Input: part model. Units: mm. Frame: model coordinates. A direction names the side the tool comes from. Coordinates: 2 decimals unless noted, no trailing zeros. Loops run counter-clockwise (first coordinate to the right, second up) from the corner with the lowest first, then second, coordinate; pieces in that order, holes last.
(1) Mould query, pull axis X, two halves, no side actions, for faces 6 (the face through (0, 4, -10)), 7 (the face through (22.5, 5, -10.1)), 8 (the face through (5, 1, -10)), 9 (the face through (45, 4, -10)). Classes: released by +X, released by -X, zero draft, split by the parting line, or undercut.
(2) Contact query for flat-ended pins moving along their axis: P1, Ø3.5, axis at x = 8, z = -8, coming from the -Y side; P2, Ø2.5, axis at x = 37.5, z = -11, coming from the -Y side. Output: stop coordinate, or through.
(3) Section B-B, the plane z = -10. Return loops of the section in (x, y), then the cut area to 3 significant figures.
(4) Set-up query: faces 1 (the face through (5, 0.5, -2.8)), 2 (the face through (2.7, 0.5, -5.5)), 3 (the face through (44.715, 0.301, -17.288)), 4 (the face through (24, 1, -14.5)), 5 (the face through (29, 0, -17)). Return all of +Z, -Z, +X, -X, +Y, -Y with unobstructed straight access to the full face (end or side cutting, diameter ignored); none if empty.
(5) Section C-C, the plane x = 8.5. Return loops of the section in (y, z), then the cut area to 3 significant figures.
(6) Section A-A, the plane y = 5. Return loops of the section in (x, z).
(7) Line query: L1, parallel to Z at x = 23.5, y = 1.75; L2, parallel to Z at x = 6.5, y = 7; L3, parallel to X at y = 5.25, z = -7. Output: solid intervals per line, ascending.
```python
from build123d import *
from OCP.BRepFilletAPI import BRepFilletAPI_MakeChamfer

# Parameters (mm, degrees)
SKETCH_1_W          = 45
SKETCH_1_H          = 20
EXTRUDE_1_DEPTH     = 8
CUT_EXTRUDE_1_DEPTH = 2
CUT_EXTRUDE_2_DEPTH = 1
CHAMFER_1_SIZE      = 1
CHAMFER_2_SIZE      = 1
CHAMFER_2_SIZE_2    = 1.732050808
FILLET_1_R          = 1


with BuildPart() as part:
    # 草图1 → 凸台-拉伸1 (new body)
    with BuildSketch(Plane(origin=(0, 0, 0), x_dir=(1, 0, 0), z_dir=(0, 1, 0))):
        with Locations((22.5, 10)):
            Rectangle(SKETCH_1_W, SKETCH_1_H)
        with BuildLine():
            Line((18, 5.5), (10, 5.5))
            ThreePointArc((10, 5.5), (5.5, 10), (10, 14.5))
            Line((10, 14.5), (18, 14.5))
            ThreePointArc((18, 14.5), (22.5, 10), (18, 5.5))
        make_face(mode=Mode.SUBTRACT)
    extrude(amount=EXTRUDE_1_DEPTH)

    # 草图2 → 切除-拉伸1 (cut)
    with BuildSketch(Plane.XZ):
        with BuildLine():
            Line((45, -5.5), (45, -14.5))
            Line((45, -14.5), (10, -14.5))
            ThreePointArc((10, -14.5), (5.5, -10), (10, -5.5))
            Line((10, -5.5), (45, -5.5))
        make_face()
    extrude(amount=-CUT_EXTRUDE_1_DEPTH, mode=Mode.SUBTRACT)

    # 草图3 → 切除-拉伸2 (cut)
    with BuildSketch(Plane.XZ):
        Polygon((0, -5.5), (5.5, -5.5), (5.5, 0), (12.1, 0), (12.1, -20), (5.5, -20), (5.5, -14.5), (0, -14.5), align=None)
    extrude(amount=-CUT_EXTRUDE_2_DEPTH, mode=Mode.SUBTRACT)

    # 倒角1
    chamfer_1_edges = [part.edges().sort_by_distance(p)[0] for p in [
        (0, 0, -17.25),
        (5.5, 0, -17.25),
        (5.5, 0, -2.75),
        (0, 0, -2.75),
    ]]
    chamfer(chamfer_1_edges, length=CHAMFER_1_SIZE - 0.0001)  # a hair under: the kernel refuses the full size

    # 倒角2
    chamfer_2_edges_1 = [part.edges().sort_by_distance(p)[0] for p in [
        (12.1, 0, -17.25),
    ]]
    chamfer_2_side_1 = [part.faces().sort_by_distance(p)[0] for p in [
        (12.1, 0.02, -17.25),
    ]]
    chamfer_2_edges_2 = [part.edges().sort_by_distance(p)[0] for p in [
        (12.1, 0, -2.75),
    ]]
    chamfer_2_side_2 = [part.faces().sort_by_distance(p)[0] for p in [
        (12.1, 0.02, -2.75),
    ]]
    chamfer_2 = BRepFilletAPI_MakeChamfer(part.part.solid().wrapped)
    for e in chamfer_2_edges_1:
        chamfer_2.Add(CHAMFER_2_SIZE - 0.0001, CHAMFER_2_SIZE_2 - 0.0001, e.wrapped, chamfer_2_side_1[0].wrapped)
    for e in chamfer_2_edges_2:
        chamfer_2.Add(CHAMFER_2_SIZE - 0.0001, CHAMFER_2_SIZE_2 - 0.0001, e.wrapped, chamfer_2_side_2[0].wrapped)
    add(Compound.cast(chamfer_2.Shape()), mode=Mode.REPLACE)  # a hair under: the kernel refuses the full size

    # 圆角1
    fillet_1_edges = [part.edges().sort_by_distance(p)[0] for p in [
        (22.5, 8, -20),
        (45, 8, -10),
        (22.5, 8, 0),
        (0, 8, -10),
        (45, 4, 0),
        (45, 4, -20),
        (0, 4.49995, -20),
        (0, 4.49995, 0),
        (45, 0, -17.25),
        (45, 0, -2.75),
    ]]
    fillet(fillet_1_edges, radius=FILLET_1_R)


solid = part.part
```
Report:
1. face 6: released by -X
1. face 7: undercut
1. face 8: undercut
1. face 9: released by +X
2. P1: stops at y = 1
2. P2: stops at y = 2
3. outline: (0, 1) - (5.5, 1) - (5.5, 8) - (1, 8) arc R1 ccw to (0, 7) - close; (22.5, 2) - (45, 2) - (45, 7) arc R1 ccw to (44, 8) - (22.5, 8) - close
3. area: 173 mm2
4. face 1: +Z, -Z, -Y
4. face 2: +X, -X, -Y
4. face 3: +Z, -Z, +X, -Y
4. face 4: -Y
4. face 5: +Z, -Z, +X, -X, -Y
5. outline: (1, -20) - (7, -20) arc R1 ccw to (8, -19) - (8, -14.24) - (1, -14.24) - close; (1, -5.76) - (8, -5.76) - (8, -1) arc R1 ccw to (7, 0) - (1, 0) - close
5. area: 80.2 mm2
6. outline: (0, -19) arc R1 ccw to (1, -20) - (44, -20) arc R1 ccw to (45, -19) - (45, -1) arc R1 ccw to (44, 0) - (1, 0) arc R1 ccw to (0, -1) - close; hole (10, -14.5) - (18, -14.5) arc R4.5 ccw to (18, -5.5) - (10, -5.5) arc R4.5 ccw to start
7. L1: z = -20 to -14.5, -5.5 to 0
7. L2: z = -20 to -12.83, -7.17 to 0
7. L3: x = 0 to 6.65, 21.35 to 45
